Source: CAD feature listing. Evaluate the final solid. Frame: model axes, mm. A direction names the side the tool comes from. Round coordinates to 2 decimals unless told otherwise and drop trailing zeros. Order: outer loops, then holes, each group sorted by start corner. A loop starts at its lowest first (then second) coordinate and runs counter-clockwise, first axis right, second up. Notation, with made-up numbers: M 51.5,79 L 93.5,79 A25 ccw 93.5,102 Z; hole C 63,-0.75 d4. An arc over 180 degrees is marked long. Answer as CSV lines item,"result". Start each with the question number.
Item 1: Section query B-B on y = -4.75. Return the cut outline in (x, z), plus the area to 3 significant figures.
Item 2: Set-up query: faces 4 (the face through (0, 10, -1)), 5 (the face through (7, 6, -0.5)). Return all of +Z, -Z, +X, -X, +Y, -Y with unobstructed straight access to the full face (end or side cutting, diameter ignored); none if empty.
Item 3: Section query C-C on z = 1.75. Return the cut outline in (x, y), plus the area to 3 significant figures.
Item 4: Pull-direction query (X, two-part tool) for faces 1 (the face through (-9.715, -9.699, -1.232)), 2 (the face through (-7, -5, 5.3)), 3 (the face through (-7, 6, -0.5)); classes: +X half, -X half, draft (parallel to the pull), parting line (faces both ways), or undercut.
Item 5: First-contact query: P1, Ø4.5, axis at x = 6.5, y = 5, coming from the +Z side; P2, Ø3, axis at x = 3.5, y = -2, coming from the +Z side. Flat tips, straight axial feed; report the tip coordinate or a pass-through.
Item 6: Section query D-D on x = -8.5. Return the cut outline in (y, z), plus the area to 3 significant figures.
Item 7: Section query A-A on x = 7. Return the cut outline in (y, z).
Item 8: Line query: line 1 (Y direction, x = -7, z = -0.4); line 2 (X direction, y = -4.75, z = -0.25); line 3 (Y direction, x = -6.5, z = 0.5). Output: solid intervals per line, ascending. Write a range as [from, to].
from build123d import *

# Parameters (mm, degrees)
BOSS_EXTRUDE1_DEPTH = 2.5
SKETCH2_W           = 0.5
SKETCH2_H           = 2
SKETCH3_W           = 0.5
SKETCH3_H           = 2
SKETCH4_W           = 0.5
SKETCH4_H           = 2
SKETCH5_W           = 0.5
SKETCH5_H           = 2


with BuildPart() as part:
    # Sketch1 → Boss-Extrude1 (new body)
    with BuildSketch(Plane.XY):
        with BuildLine():
            Line((-10, 9), (-10, -9))
            ThreePointArc((-10, -9), (-9.707106781, -9.707106781), (-9, -10))
            Line((-9, -10), (9, -10))
            ThreePointArc((9, -10), (9.707106781, -9.707106781), (10, -9))
            Line((10, -9), (10, 9))
            ThreePointArc((10, 9), (9.707106781, 9.707106781), (9, 10))
            Line((9, 10), (-9, 10))
            ThreePointArc((-9, 10), (-9.707106781, 9.707106781), (-10, 9))
        make_face()
    extrude(amount=-BOSS_EXTRUDE1_DEPTH)

    # Sketch2 → Cut-Revolve1 (revolve, cut)
    with BuildSketch(Plane(origin=(-7, 0, 0), x_dir=(0, 0, -1), z_dir=(1, 0, 0))):
        with Locations((0.25, 5.75)):
            Rectangle(SKETCH2_W, SKETCH2_H)
    revolve(axis=Axis((-7, 4.75, -0.5), (0, 0, 1)), mode=Mode.SUBTRACT)

    # Sketch3 → Cut-Revolve2 (revolve, cut)
    with BuildSketch(Plane(origin=(7, 0, 0), x_dir=(0, 0, -1), z_dir=(1, 0, 0))):
        with Locations((0.25, 5.75)):
            Rectangle(SKETCH3_W, SKETCH3_H)
    revolve(axis=Axis((7, 4.75, -0.5), (0, 0, 1)), mode=Mode.SUBTRACT)

    # Sketch4 → Cut-Revolve3 (revolve, cut)
    with BuildSketch(Plane(origin=(7, 0, 0), x_dir=(0, 0, -1), z_dir=(1, 0, 0))):
        with Locations((0.25, -3.75)):
            Rectangle(SKETCH4_W, SKETCH4_H)
    revolve(axis=Axis((7, -4.75, -0.5), (0, 0, 1)), mode=Mode.SUBTRACT)

    # Sketch5 → Cut-Revolve4 (revolve, cut)
    with BuildSketch(Plane(origin=(-7, 0, 0), x_dir=(0, 0, -1), z_dir=(1, 0, 0))):
        with Locations((0.25, -3.75)):
            Rectangle(SKETCH5_W, SKETCH5_H)
    revolve(axis=Axis((-7, -4.75, -0.5), (0, 0, 1)), mode=Mode.SUBTRACT)

    # Sketch6 → Revolve1 (revolve)
    with BuildSketch(Plane(origin=(-7, 0, 0), x_dir=(0, 0, -1), z_dir=(1, 0, 0))):
        Polygon((-5.3, 4.75), (-5.3, 5.25), (-3.8, 5.75), (0.5, 5.75), (0.5, 4.75), align=None)
    revolve(axis=Axis((-7, 4.75, -0.5), (0, 0, 1)))

    # Sketch7 → Revolve2 (revolve)
    with BuildSketch(Plane(origin=(7, 0, 0), x_dir=(0, 0, -1), z_dir=(1, 0, 0))):
        Polygon((-5.3, 4.75), (-5.3, 5.25), (-3.8, 5.75), (0.5, 5.75), (0.5, 4.75), align=None)
    revolve(axis=Axis((7, 4.75, -0.5), (0, 0, 1)))

    # Sketch8 → Revolve3 (revolve)
    with BuildSketch(Plane(origin=(7, 0, 0), x_dir=(0, 0, -1), z_dir=(1, 0, 0))):
        Polygon((-5.3, -4.75), (-5.3, -4.25), (-3.8, -3.75), (0.5, -3.75), (0.5, -4.75), align=None)
    revolve(axis=Axis((7, -4.75, -0.5), (0, 0, 1)))

    # Sketch9 → Revolve4 (revolve)
    with BuildSketch(Plane(origin=(-7, 0, 0), x_dir=(0, 0, -1), z_dir=(1, 0, 0))):
        Polygon((-5.3, -4.75), (-5.3, -4.25), (-3.8, -3.75), (0.5, -3.75), (0.5, -4.75), align=None)
    revolve(axis=Axis((-7, -4.75, -0.5), (0, 0, 1)))


solid = part.part
Results:
1,outline,"M -10,-2.5 L 10,-2.5 L 10,0 L 9,0 L 9,-0.5 L 8,-0.5 L 8,3.8 L 7.5,5.3 L 6.5,5.3 L 6,3.8 L 6,-0.5 L 5,-0.5 L 5,0 L -5,0 L -5,-0.5 L -6,-0.5 L -6,3.8 L -6.5,5.3 L -7.5,5.3 L -8,3.8 L -8,-0.5 L -9,-0.5 L -9,0 L -10,0 Z"
1,area,"67.7 mm^2"
2,face 4,"+Z, -Z, +X, -X, +Y"
2,face 5,"+Z"
3,outline,"C -7,-4.75 d2; C -7,4.75 d2; C 7,-4.75 d2; C 7,4.75 d2"
3,area,"12.6 mm^2"
4,face 1,"-X half"
4,face 2,"draft"
4,face 3,"undercut"
5,P1,"z = 5.3"
5,P2,"z = 0"
6,outline,"M -10,-2.5 L 10,-2.5 L 10,0 L 6.07,0 L 6.07,-0.5 L 3.43,-0.5 L 3.43,0 L -3.43,0 L -3.43,-0.5 L -6.07,-0.5 L -6.07,0 L -10,0 Z"
6,area,"47.4 mm^2"
7,outline,"M -10,-2.5 L 10,-2.5 L 10,0 L 6.75,0 L 6.75,-0.5 L 5.75,-0.5 L 5.75,3.8 L 5.25,5.3 L 4.25,5.3 L 3.75,3.8 L 3.75,-0.5 L 2.75,-0.5 L 2.75,0 L -2.75,0 L -2.75,-0.5 L -3.75,-0.5 L -3.75,3.8 L -4.25,5.3 L -5.25,5.3 L -5.75,3.8 L -5.75,-0.5 L -6.75,-0.5 L -6.75,0 L -10,0 Z"
8,line 1,"[-10, -6.75], [-5.75, -3.75], [-2.75, 2.75], [3.75, 5.75], [6.75, 10]"
8,line 2,"[-10, -9], [-8, -6], [-5, 5], [6, 8], [9, 10]"
8,line 3,"[-5.62, -3.88], [3.88, 5.62]"
